from build123d import *

# Parameters (mm, degrees)
F0_W     = 693
F0_H     = 131.4
F0_R     = 1.575
F0_W_2   = 37.74
F0_H_2   = 32.26
F0_R_2   = 3.25
F0_W_3   = 27.43
F0_H_3   = 27.43
F0_W_4   = 43.13
F0_H_4   = 43.13
F1_DEPTH = 2


with BuildPart() as f1:
    # F0 (on Top) → F1 (new body)
    with BuildSketch(Plane.XY):
        with Locations((20.0601496525, -52.194238013)):
            Rectangle(F0_W, F0_H)
        with Locations((-302.4398503475, -109.894238013)):
            Circle(F0_R, mode=Mode.SUBTRACT)
        with Locations((-239.4398503475, -77.044238013)):
            Rectangle(F0_W_2, F0_H_2, mode=Mode.SUBTRACT)
        with Locations((-158.5898503475, -77.044238013)):
            Rectangle(F0_W_2, F0_H_2, mode=Mode.SUBTRACT)
        with Locations((-98.8898503475, -77.044238013)):
            Rectangle(F0_W_2, F0_H_2, mode=Mode.SUBTRACT)
        with Locations((-39.1898503475, -77.044238013)):
            Rectangle(F0_W_2, F0_H_2, mode=Mode.SUBTRACT)
        with Locations((187.1601496525, -89.469238013)):
            Circle(F0_R_2, mode=Mode.SUBTRACT)
        with Locations((342.5601496525, -109.894238013)):
            Circle(F0_R, mode=Mode.SUBTRACT)
        with Locations((20.5101496525, -77.044238013)):
            Rectangle(F0_W_2, F0_H_2, mode=Mode.SUBTRACT)
        with Locations((80.2101496525, -77.044238013)):
            Rectangle(F0_W_2, F0_H_2, mode=Mode.SUBTRACT)
        with Locations((187.1601496525, -65.7151937485)):
            Circle(F0_R_2, mode=Mode.SUBTRACT)
        with Locations((243.5601496525, -77.044238013)):
            Rectangle(F0_W_3, F0_H_3, mode=Mode.SUBTRACT)
        with Locations((284.5601496525, -77.044238013)):
            Rectangle(F0_W_3, F0_H_3, mode=Mode.SUBTRACT)
        with Locations((-264.9398503475, -27.344238013)):
            Rectangle(F0_W_3, F0_H_3, mode=Mode.SUBTRACT)
        with Locations((-213.9398503475, -27.344238013)):
            Rectangle(F0_W_3, F0_H_3, mode=Mode.SUBTRACT)
        with Locations((-158.5898503475, -27.344238013)):
            Rectangle(F0_W_2, F0_H_2, mode=Mode.SUBTRACT)
        with Locations((-98.8898503475, -27.344238013)):
            Rectangle(F0_W_2, F0_H_2, mode=Mode.SUBTRACT)
        with Locations((-39.1898503475, -27.344238013)):
            Rectangle(F0_W_2, F0_H_2, mode=Mode.SUBTRACT)
        with Locations((-302.4398503475, 5.505761987)):
            Circle(F0_R, mode=Mode.SUBTRACT)
        with Locations((143.4101496525, -52.194238013)):
            Rectangle(F0_W_4, F0_H_4, mode=Mode.SUBTRACT)
        with Locations((187.1601496525, -40.0840714574)):
            Circle(F0_R_2, mode=Mode.SUBTRACT)
        with Locations((20.5101496525, -27.344238013)):
            Rectangle(F0_W_2, F0_H_2, mode=Mode.SUBTRACT)
        with Locations((80.2101496525, -27.344238013)):
            Rectangle(F0_W_2, F0_H_2, mode=Mode.SUBTRACT)
        with Locations((223.0601496525, -27.344238013)):
            Rectangle(F0_W_3, F0_H_3, mode=Mode.SUBTRACT)
        with Locations((264.0601496525, -27.344238013)):
            Rectangle(F0_W_3, F0_H_3, mode=Mode.SUBTRACT)
        with Locations((305.0601496525, -27.344238013)):
            Rectangle(F0_W_3, F0_H_3, mode=Mode.SUBTRACT)
        with Locations((187.1601496525, -14.919238013)):
            Circle(F0_R_2, mode=Mode.SUBTRACT)
        with Locations((342.5601496525, 5.505761987)):
            Circle(F0_R, mode=Mode.SUBTRACT)
    extrude(amount=F1_DEPTH)


solid = f1.part
Verification items for the finished model (mm, model axes). Coordinates: 2 decimals unless noted, no trailing zeros. Order: outer loops, then holes, each group sorted by start corner. A loop starts at its lowest first (then second) coordinate and runs counter-clockwise, first axis right, second up. Notation, with made-up numbers: M 25.25,-35 L 51.25,-35 A18 ccw 51.25,-18 Z; hole C 23,31.25 d8. An arc over 180 degrees is marked long. One line per item, written item: value. Start each with the question number.
Item 1: Sectioned sample at C-C on z = 0.9. Give the number of separate pieces and of enclosed holes in the cut face, then the cut area to 3 significant figures.
Item 2: Depth check by flat-ended pin: P1, Ø6, axis at x = 187.16, y = -14.92, coming from the -Z side. Enter the tip coordinate at first touch or a pass-through.
Item 3: Thickness scan on probe 1 along Y at (x, z) = (-55, 1.1); probe 2 along Y at (x, z) = (-222.5, 1.6); probe 3 along Y at (x, z) = (-213, 0.55). Record the ranges inside material, lowest first.
Item 4: Sectioned sample at A-A on x = -235.5. Record the cut outline in (y, z).
Item 5: Sectioned sample at B-B on x = -156.5. Record the cut outline in (y, z).
Calculated:
1. separate pieces: 1
1. enclosed holes: 27
1. area: 70,400 mm^2
2. P1: through
3. probe 1: -117.89 to -93.17, -60.91 to -43.47, -11.21 to 13.51
3. probe 2: -117.89 to -93.17, -60.91 to -41.06, -13.63 to 13.51
3. probe 3: -117.89 to -41.06, -13.63 to 13.51
4. outline: M -117.89,0 L -93.17,0 L -93.17,2 L -117.89,2 Z; M -60.91,0 L 13.51,0 L 13.51,2 L -60.91,2 Z
5. outline: M -117.89,0 L -93.17,0 L -93.17,2 L -117.89,2 Z; M -60.91,0 L -43.47,0 L -43.47,2 L -60.91,2 Z; M -11.21,0 L 13.51,0 L 13.51,2 L -11.21,2 Z
